Build history of the part. All positions in model axes, mm. Coordinates: 2 decimals unless noted, no trailing zeros. Loops run counter-clockwise (first coordinate to the right, second up) from the corner with the lowest first, then second, coordinate; pieces in that order, holes last.
(1) Slice it at B-B (z = 26.5). Give the cut face in (x, y) (3 decimals).
(2) Slice it at A-A (x = 0). Give the cut face in (y, z) (3 decimals).
(3) Slice it at C-C (z = 91.5). Give the cut face in (x, y) (3 decimals).
(4) Wall check: L1, parallel to Y at x = -0.3, z = 56.5; L2, parallel to Y at x = 0.25, z = 53; L3, parallel to Y at x = -0.45, z = 34. Give the ranges that are in metal, low to high.
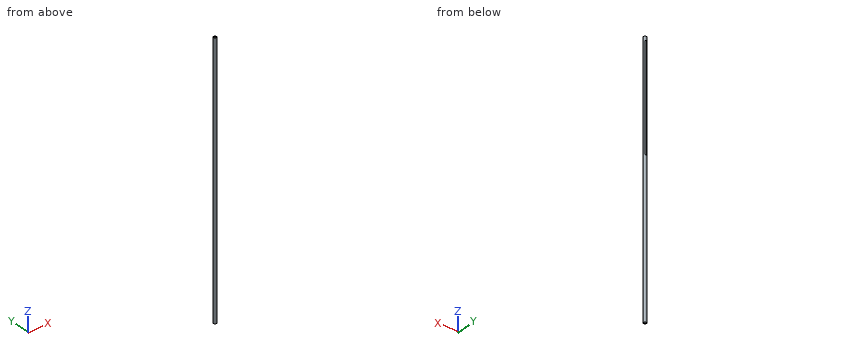
from build123d import *

# Parameters (mm, degrees)
SKETCH1_R           = 0.535
SKETCH1_R_2         = 0.405
BOSS_EXTRUDE1_DEPTH = 100
SKETCH2_W           = 0.7
SKETCH2_H           = 40
CUT_EXTRUDE1_DEPTH  = 1.535


with BuildPart() as part:
    # Sketch1 → Boss-Extrude1 (new body)
    with BuildSketch(Plane.XY):
        Circle(SKETCH1_R)
        Circle(SKETCH1_R_2, mode=Mode.SUBTRACT)
    extrude(amount=BOSS_EXTRUDE1_DEPTH)

    # Sketch2 → Cut-Extrude1 (cut, through all)
    with BuildSketch(Plane(origin=(0, 0, 0), x_dir=(1, 0, 0), z_dir=(0, 1, 0))):
        with Locations((0, -78.5)):
            Rectangle(SKETCH2_W, SKETCH2_H)
    extrude(amount=CUT_EXTRUDE1_DEPTH, mode=Mode.SUBTRACT)


solid = part.part
Response values:
1. outline: circle Ø1.07 at (0, 0); hole circle Ø0.81 at (0, 0)
2. outline: (-0.535, 0) - (-0.405, 0) - (-0.405, 100) - (-0.535, 100) - close; (0.405, 0) - (0.535, 0) - (0.535, 58.5) - (0.405, 58.5) - close; (0.405, 98.5) - (0.535, 98.5) - (0.535, 100) - (0.405, 100) - close
3. outline: (-0.35, 0.204) - (-0.35, 0.405) arc R0.535 ccw (long way) to (0.35, 0.405) - (0.35, 0.204) arc R0.405 cw (long way) to start
4. L1: y = -0.44 to -0.27, 0.27 to 0.44
4. L2: y = -0.47 to -0.32, 0.32 to 0.47
4. L3: y = -0.29 to 0.29
